Here's the drawing with two shaded views (mm, measured from the low corner). I have some questions. A direction names the side the tool comes from. Round coordinates to 2 decimals unless told otherwise and drop trailing zeros. Loops run counter-clockwise (first coordinate to the right, second up) from the corner with the lowest first, then second, coordinate; pieces in that order, holes last. Notation, with made-up numbers: (81.5, 77.25) -> (89.5, 77.25) arc R16 ccw to (89.5, 102.25) -> close; hole circle Ø11 at (60.25, 24). An arc over 180 degrees is marked (long way). Write each question's results on one line, items separated by ' | '. Start each with the question number.
1) Which directions (+Z, -Z, +X, -X, +Y, -Y) give clear straight access to the entire face, cutting with the end or side of a thin tool? Please do the marked faces 1 and 2.
2) For P1, Ø7.5, axis at x = 12.7, y = 12.7, coming from the +Z side, with a flat end and sliding along its axis, tell me the tip position at first contact or that it passes through.
3) Imagine slicing it at C-C, the plane x = 4.75. List the corners of the cut face in (y, z) for me.
4) We'd pull the mould along Z, two halves only. Please class the marked faces 3, 4 and 5: pulls with the +Z half, pulls with the -Z half, needs draft (parallel to the pull), parting line crosses it, or undercut.
5) Imagine slicing it at A-A, the plane x = 12.7. List the corners of the cut face in (y, z) for me.
6) If I drill on probe 1 along Y at (x, z) = (0.8, 12.7); probe 2 along Y at (x, z) = (12.7, 24.45); probe 3 along Z at (x, y) = (17.5, 110), over which ranges is the centre line in solid material (lowest first)?
7) Imagine slicing it at B-B, the plane y = 25.4. List the corners of the cut face in (x, z) for me, plus the area to 3 significant figures.
8) Imagine slicing it at D-D, the plane z = 16.5. List the corners of the cut face in (x, y) for me.
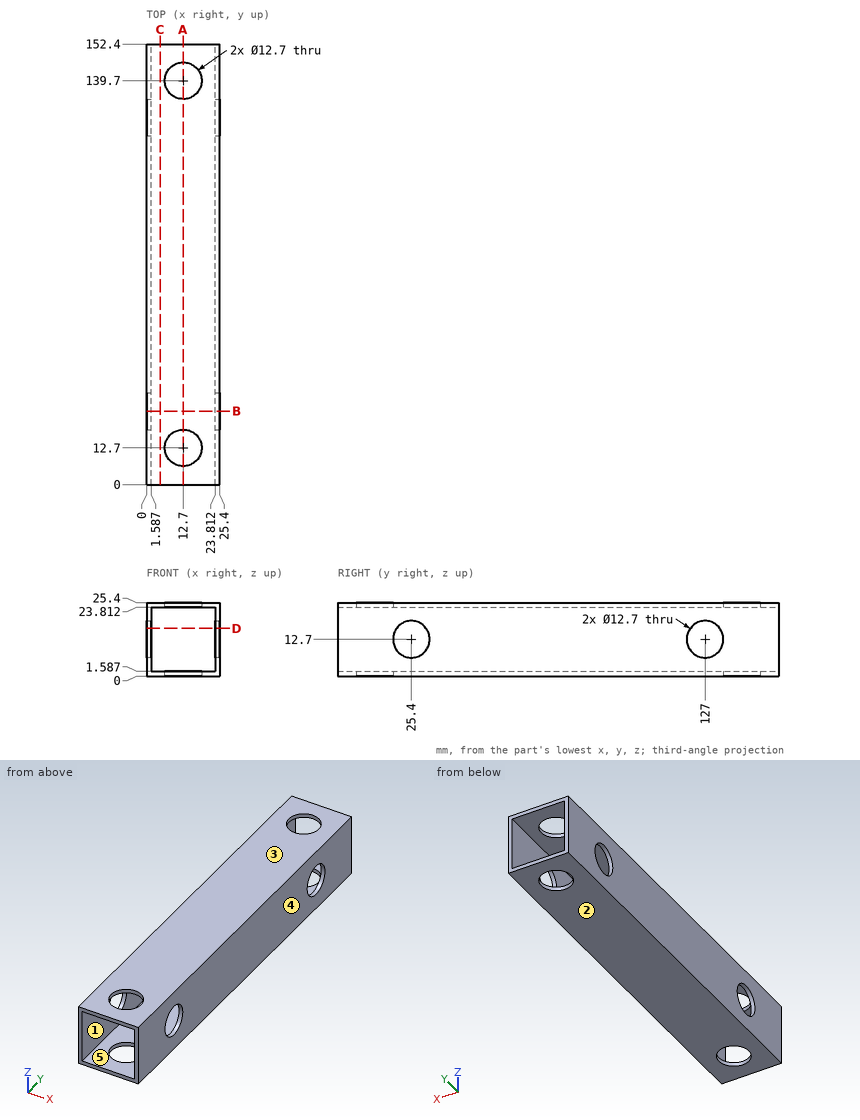
Checked values:
1) face 1: +Y, -Y | face 2: -Z, +X, -X, +Y, -Y
2) P1: through
3) outline: (0, 0) -> (152.4, 0) -> (152.4, 1.59) -> (0, 1.59) -> close; (0, 23.81) -> (152.4, 23.81) -> (152.4, 25.4) -> (0, 25.4) -> close
4) face 3: pulls with the +Z half | face 4: needs draft | face 5: undercut
5) outline: (0, 0) -> (6.35, 0) -> (6.35, 1.59) -> (0, 1.59) -> close; (0, 23.81) -> (6.35, 23.81) -> (6.35, 25.4) -> (0, 25.4) -> close; (19.05, 0) -> (133.35, 0) -> (133.35, 1.59) -> (19.05, 1.59) -> close; (19.05, 23.81) -> (133.35, 23.81) -> (133.35, 25.4) -> (19.05, 25.4) -> close; (146.05, 0) -> (152.4, 0) -> (152.4, 1.59) -> (146.05, 1.59) -> close; (146.05, 23.81) -> (152.4, 23.81) -> (152.4, 25.4) -> (146.05, 25.4) -> close
6) probe 1: 0 to 19.05, 31.75 to 120.65, 133.35 to 152.4 | probe 2: 0 to 6.35, 19.05 to 133.35, 146.05 to 152.4 | probe 3: 0 to 1.59, 23.81 to 25.4
7) outline: (0, 0) -> (25.4, 0) -> (25.4, 6.35) -> (23.81, 6.35) -> (23.81, 1.59) -> (1.59, 1.59) -> (1.59, 6.35) -> (0, 6.35) -> close; (0, 19.05) -> (1.59, 19.05) -> (1.59, 23.81) -> (23.81, 23.81) -> (23.81, 19.05) -> (25.4, 19.05) -> (25.4, 25.4) -> (0, 25.4) -> close | area: 111 mm^2
8) outline: (0, 0) -> (1.59, 0) -> (1.59, 20.31) -> (0, 20.31) -> close; (0, 30.49) -> (1.59, 30.49) -> (1.59, 121.91) -> (0, 121.91) -> close; (0, 132.09) -> (1.59, 132.09) -> (1.59, 152.4) -> (0, 152.4) -> close; (23.81, 0) -> (25.4, 0) -> (25.4, 20.31) -> (23.81, 20.31) -> close; (23.81, 30.49) -> (25.4, 30.49) -> (25.4, 121.91) -> (23.81, 121.91) -> close; (23.81, 132.09) -> (25.4, 132.09) -> (25.4, 152.4) -> (23.81, 152.4) -> close
